Can you work these out from the drawing? Everything is in mm from the part's minimum corner. Coordinates: 2 decimals unless noted, no trailing zeros. Loops run counter-clockwise (first coordinate to the right, second up) from the corner with the lowest first, then second, coordinate; pieces in that order, holes last.
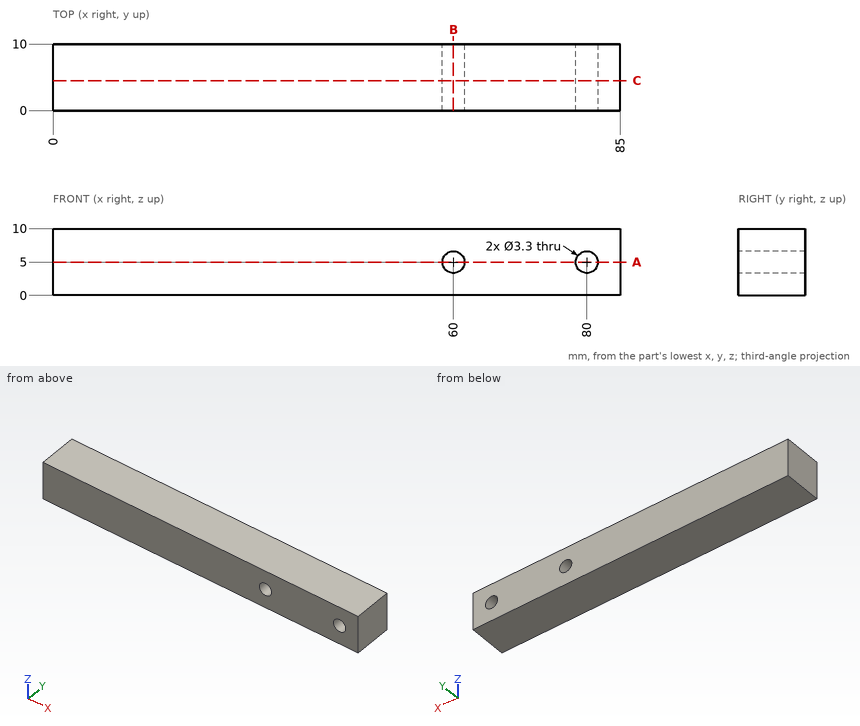
Item 1: Suppose I cut it at C-C, the plane y = 4.5. Please give me the cut outline in (x, z), plus the area to 3 significant figures.
Results are:
outline: (0, 0) - (85, 0) - (85, 10) - (0, 10) - close; hole circle Ø3.3 at (60, 5); hole circle Ø3.3 at (80, 5)
area: 833 mm2
Item 2: Suppose I cut it at A-A, the plane z = 5. Please give me the cut outline in (x, y).
Results are:
outline: (0, 0) - (58.35, 0) - (58.35, 10) - (0, 10) - close; (61.65, 0) - (78.35, 0) - (78.35, 10) - (61.65, 10) - close; (81.65, 0) - (85, 0) - (85, 10) - (81.65, 10) - close
Item 3: I need wall thicknesses on line 1 along Z through (x, y) = (80, 5); line 2 along X through (y, z) = (3.25, 4.25); line 3 along X through (y, z) = (2.5, 6). Which ranges of each line are inside material? Lowest first, please.
Results are:
line 1: z = 0 to 3.35, 6.65 to 10
line 2: x = 0 to 58.53, 61.47 to 78.53, 81.47 to 85
line 3: x = 0 to 58.69, 61.31 to 78.69, 81.31 to 85
Item 4: Suppose I cut it at B-B, the plane x = 60. Please give me the cut outline in (y, z).
Results are:
outline: (0, 0) - (10, 0) - (10, 3.35) - (0, 3.35) - close; (0, 6.65) - (10, 6.65) - (10, 10) - (0, 10) - close
